Autodesk Inventor part; units mm, degrees
ref_plane "Flange Pattern Plane" through (19.05, 7.9375, -4.5466) normal (0, 1, 0) x (1, 0, 0)
ref_plane "YZ Plane" through (0, 0, 0) normal (1, 0, 0) x (0, 1, 0)
ref_plane "XZ Plane" through (0, 0, 0) normal (0, 1, 0) x (-1, 0, 0)
sketch "Sketch1" plane through (0, 0, 0) normal (0, 1, 0) x (-1, 0, 0)
  line L0 (-19.05, 0) -> (19.05, 0)
  line L1 (19.05, 0) -> (19.05, -12.7)
  line L2 (19.05, -12.7) -> (-19.05, -12.7)
  line L3 (-19.05, -12.7) -> (-19.05, 0)
  line L4 (19.05, 0) -> (-19.05, -12.7) construction
  point P0 (0, 0)
  point P1 (0, 0)
  dimension "d0" = 38.1
  dimension "d1" = 12.7
extrude "Plate1" add sketch "Sketch1" along normal blind 1.5875
sketch "Sketch2" plane through (17.4625, 0, -12.7) normal (1, 0, 0) x (0, 1, 0)
  line L0 (0, 12.7) -> (0, 0)
  line L1 (0, 0) -> (14.2875, 0)
  line L2 (14.2875, 0) -> (14.2875, 12.7)
  line L3 (14.2875, 12.7) -> (0, 12.7)
edge flange "Flanges" height 12.7 angle 90 thickness 1.5875 bend radius 0.7937 thickness toward (1, 0, 0) relief tear relief width 1.5875 relief depth 0.7937 corner gap 1.5875 corner form 0 edges at (19.05, 1.5875, -6.35) (-19.05, 1.5875, -6.35) wall of the first edge with corners at (17.4625, 0, 0) (17.4625, 0, -12.7) (17.4625, 14.2875, -12.7) (17.4625, 14.2875, 0)
bend "Bend1"
corner "Corner1"
sketch "Sketch3" plane through (19.05, 2.3813, -12.7) normal (1, 0, 0) x (0, 0, -1)
  line L0 (-8.1534, 7.8676) -> (-4.5466, 7.8676)
  line L1 (-4.0386, 7.3596) -> (-4.0386, 3.7529)
  line L2 (-4.5466, 3.2449) -> (-8.1534, 3.2449)
  line L3 (-8.6614, 3.7529) -> (-8.6614, 7.3596)
  arc A0 (-8.1534, 7.8676) -> (-8.6614, 7.3596) centre (-8.1534, 7.3596) ccw
  arc A1 (-4.0386, 7.3596) -> (-4.5466, 7.8676) centre (-4.5466, 7.3596) ccw
  arc A2 (-4.5466, 3.2449) -> (-4.0386, 3.7529) centre (-4.5466, 3.7529) ccw
  arc A3 (-8.6614, 3.7529) -> (-8.1534, 3.2449) centre (-8.1534, 3.7529) ccw
  line L4 (-12.7, 0) -> (-12.7, 11.9063) construction
  line L5 (-12.7, 11.9063) -> (0, 11.9063) construction
  line L6 (-8.1534, 7.3596) -> (-4.5466, 3.7529) construction
  point P0 (-12.7, -2.3812)
  point P1 (-4.0386, 3.2449)
  point P2 (-8.6614, 3.2449)
  point P3 (-6.35, 5.5563)
  dimension "d16" = 4.6228
  dimension "d17" = 0.508
  dimension "d20" = 6.35
  dimension "d21" = 6.35
extrude "Flange Stamp" cut sketch "Sketch3" against normal blind 1.5875
sketch "Sketch7" plane through (19.05, 2.3813, 0) normal (1, 0, 0) x (0, 0, -1)
  arc A0 (4.5466, 7.8676) -> (4.0386, 7.3596) centre (4.5466, 7.3596) ccw construction
  arc A1 (8.1534, 3.2449) -> (8.6614, 3.7529) centre (8.1534, 3.7529) ccw construction
  circle A2 centre (6.35, 5.5563) radius 2.1844
  line L0 (4.5466, 7.3596) -> (8.1534, 3.7529) construction
  point P0 (0, -2.3812)
  dimension "d46" = 4.3688
surface extrude "Flange Circle" sketch "Sketch7" against normal up to surface (1.5875 mm away) shown yes curves A2
ref_plane "Flange Pattern Plane" through (19.05, 7.9375, -4.5466) normal (0, 1, 0) x (1, 0, 0)
feature "Flange Pattern" [suppressed]
sketch "Sketch8" plane through (0, 0, 0) normal (0, -1, 0) x (1, 0, 0)
  line L0 (16.6687, 0) -> (-16.6687, 0) construction
  line L1 (14.5034, -4.0386) -> (10.8966, -4.0386)
  line L2 (10.3886, -4.5466) -> (10.3886, -8.1534)
  line L3 (10.8966, -8.6614) -> (14.5034, -8.6614)
  line L4 (15.0114, -8.1534) -> (15.0114, -4.5466)
  arc A0 (15.0114, -4.5466) -> (14.5034, -4.0386) centre (14.5034, -4.5466) ccw
  arc A1 (14.5034, -8.6614) -> (15.0114, -8.1534) centre (14.5034, -8.1534) ccw
  arc A2 (10.3886, -8.1534) -> (10.8966, -8.6614) centre (10.8966, -8.1534) ccw
  arc A3 (10.8966, -4.0386) -> (10.3886, -4.5466) centre (10.8966, -4.5466) ccw
  line L5 (14.5034, -4.5466) -> (10.8966, -8.1534) construction
  line L6 (19.05, 0) -> (19.05, -12.7) construction
  point P0 (0, 0)
  point P1 (10.3886, -8.6614)
  point P2 (15.0114, -8.6614)
  point P3 (12.7, -6.35)
  dimension "d49" = 4.6228
  dimension "d50" = 0.508
  dimension "d51" = 6.35
  dimension "d52" = 6.35
extrude "Body Stamp" cut sketch "Sketch8" against normal blind 1.5875
sketch "Sketch9" plane through (0, 0, 0) normal (0, -1, 0) x (1, 0, 0)
  arc A0 (15.0114, -4.5466) -> (14.5034, -4.0386) centre (14.5034, -4.5466) ccw construction
  arc A1 (10.3886, -8.1534) -> (10.8966, -8.6614) centre (10.8966, -8.1534) ccw construction
  line L0 (14.5034, -4.5466) -> (10.8966, -8.1534) construction
  circle A2 centre (12.7, -6.35) radius 2.1844
  point P0 (0, 0)
  dimension "d55" = 4.3688
surface extrude "Body Circle" sketch "Sketch9" against normal up to surface (1.5875 mm away) shown yes curves A2
feature "Body Pattern" [suppressed]
sketch "Arc Length" plane through (17.4625, 2.3813, 0) normal (0, 0, 1) x (1, 0, 0)
  line L0 (0, 0) -> (1.5875, 0) construction
  arc A0 (-0.7938, -0.7938) -> (0, 0) centre (-0.7937, 0) ccw construction
  line L1 (-0.7938, -2.3813) -> (-0.7938, -0.7938) construction
  arc A1 (-0.7938, -2.3813) -> (1.5875, 0) centre (-0.7937, 0) ccw construction
  point P0 (-17.4625, -2.3812)
  dimension "d85" = 3.7405
  dimension "d92" = 1.2468
sketch "Sketch13" plane through (19.05, 14.2875, 0) normal (1, 0, 0) x (0, 0, -1)
  line L0 (0, 0) -> (12.7, 0) construction
  line L1 (62.4078, 0) -> (63.4238, -1.016)
  line L2 (63.4238, -1.016) -> (64.4398, 0)
  line L3 (62.4078, 0) -> (64.4398, 0)
  line L4 (12.7, -11.9063) -> (0, -11.9062) construction
  line L5 (63.4238, -10.8903) -> (61.161, -13.1531)
  line L6 (61.161, -13.1531) -> (63.4238, -15.4159)
  line L7 (63.4238, -15.4159) -> (65.6866, -13.1531)
  line L8 (65.6866, -13.1531) -> (63.4238, -10.8903)
  line L9 (63.4238, -10.8903) -> (63.4238, -15.4159) construction
  line L10 (63.4238, -1.016) -> (63.4238, -10.8903) construction
  line L11 (0, -11.9062) -> (12.7, -11.9063) construction
  point P0 (0, -14.2875)
  dimension "d86" = 4.5256
  dimension "d88" = 1.016
  dimension "d91" = 1.016
  dimension "d102" = 63.4238
feature "Notch" [suppressed]
mirror "Notch Mirror" [suppressed]
pattern_linear "Notch Pattern" [suppressed]
chamfer "End Chamfer" distance 1.016 angle 45 4 edges at (-18.2563, 14.2875, -12.7) (18.2563, 14.2875, -12.7) (-18.2562, 14.2875, 0) (18.2562, 14.2875, 0)
sketch "Sketch14" plane through (-19.05, 2.3813, 431.8) normal (1, 0, 0) x (0, 0, -1)
  line L0 (431.8, 11.9063) -> (444.5, 11.9063) construction
  line L1 (431.8, 0) -> (431.8, 11.9063) construction
  line L2 (431.8, -2.3813) -> (444.5, -2.3813) construction
  line L3 (431.8, 11.9063) -> (444.5, 11.9063)
  line L4 (444.5, 11.9063) -> (444.5, -2.3813)
  line L5 (444.5, -2.3813) -> (431.8, -2.3813)
  line L6 (431.8, -2.3813) -> (431.8, 11.9063)
  point P0 (431.8, -2.3812)
  point P1 (382.0521, -1.9844)
extrude "Half Cut" cut sketch "Sketch14" along normal blind 25.4
sketch "Flange Pattern Sketch" plane through (19.05, 7.9375, -4.5466) normal (0, 1, 0) x (1, 0, 0)
  line L0 (0, 3.6068) -> (0, 0) construction
  line L1 (-45.8186, -4.5466) -> (8.2118, -4.5466) construction
  line L2 (0, 0) -> (-1.5875, 0) construction
  point P0 (-19.05, -4.5466)
  point P1 (0, 1.8034)
  point P2 (0, 14.5034)
  point P3 (0, 27.2034)
  point P4 (0, 39.9034)
  point P5 (0, 52.6034)
  point P6 (0, 65.3034)
  point P7 (0, 78.0034)
  point P8 (0, 90.7034)
  point P9 (0, 103.4034)
  point P10 (0, 116.1034)
  point P11 (0, 128.8034)
  point P12 (0, 141.5034)
  point P13 (0, 154.2034)
  point P14 (0, 166.9034)
  point P15 (0, 179.6034)
  point P16 (0, 192.3034)
  point P17 (0, 205.0034)
  point P18 (0, 217.7034)
  point P19 (0, 230.4034)
  point P20 (0, 243.1034)
  point P21 (0, 255.8034)
  point P22 (0, 268.5034)
  point P23 (0, 281.2034)
  point P24 (0, 293.9034)
  point P25 (0, 306.6034)
  point P26 (0, 319.3034)
  point P27 (0, 332.0034)
  point P28 (0, 344.7034)
  point P29 (0, 357.4034)
  point P30 (0, 370.1034)
  point P31 (0, 382.8034)
  point P32 (0, 395.5034)
  point P33 (0, 408.2034)
  point P34 (0, 420.9034)
  point P35 (0, 433.6034)
  dimension "d131" = 12.7
  dimension "d134" = 12.7
sketch "Body Pattern Sketch" plane through (0, 0, 0) normal (0, -1, 0) x (1, 0, 0)
  line L0 (16.6687, 0) -> (-16.6687, 0) construction
  line L1 (19.05, 0) -> (19.05, -12.7) construction
  circle A0 centre (12.7, -6.35) radius 2.1844 construction
  point P0 (0, 0)
  point P1 (12.7, -19.05)
  point P2 (12.7, -31.75)
  point P3 (12.7, -44.45)
  point P4 (12.7, -57.15)
  point P5 (12.7, -69.85)
  point P6 (12.7, -82.55)
  point P7 (12.7, -95.25)
  point P8 (12.7, -107.95)
  point P9 (12.7, -120.65)
  point P10 (12.7, -133.35)
  point P11 (12.7, -146.05)
  point P12 (12.7, -158.75)
  point P13 (12.7, -171.45)
  point P14 (12.7, -184.15)
  point P15 (12.7, -196.85)
  point P16 (12.7, -209.55)
  point P17 (12.7, -222.25)
  point P18 (12.7, -234.95)
  point P19 (12.7, -247.65)
  point P20 (12.7, -260.35)
  point P21 (12.7, -273.05)
  point P22 (12.7, -285.75)
  point P23 (12.7, -298.45)
  point P24 (12.7, -311.15)
  point P25 (12.7, -323.85)
  point P26 (12.7, -336.55)
  point P27 (12.7, -349.25)
  point P28 (12.7, -361.95)
  point P29 (12.7, -374.65)
  point P30 (12.7, -387.35)
  point P31 (12.7, -400.05)
  point P32 (12.7, -412.75)
  point P33 (12.7, -425.45)
  point P34 (12.7, -438.15)
  dimension "d62" = 12.7
  dimension "d65" = 12.7
  dimension "d139" = 12.7
equation "\"d1\" = 1.27 * Length"
equation "\"d18\" = Thickness"
equation "\"d53\" = Thickness"
equation "\"d89\" = Thickness"
equation "\"d2\" = Thickness"
equation "\"d3\" = BendReliefWidth"
equation "\"d4\" = BendReliefDepth"
equation "\"d5\" = MinimumRemnant"
equation "\"d6\" = TransitionRadius"
equation "\"d10\" = CornerReliefSize"
equation "\"d11\" = GapSize"
equation "\"d12\" = JacobiRadiusSize"
equation "\"BendRadius\" = Thickness"
equation "\"BendReliefWidth\" = Thickness"
equation "\"BendReliefDepth\" = 0.5 * Thickness"
equation "\"CornerReliefSize\" = 4 * Thickness"
equation "\"MinimumRemnant\" = 2 * Thickness"
equation "\"TransitionRadius\" = BendRadius"
equation "\"JacobiRadiusSize\" = BendRadius"
equation "\"GapSize\" = Thickness"
properties part number "Alu C 1x3x1x35"
The listing builds one solid part. Answer for the finished solid, in the listing's coordinates (mm). A direction names the side the tool comes from. Round coordinates to 2 decimals unless told otherwise and drop trailing zeros. Order: outer loops, then holes, each group sorted by start corner. A loop starts at its lowest first (then second) coordinate and runs counter-clockwise, first axis right, second up. Notation, with made-up numbers: (89, -12.5) -> (119, -12.5) arc R36 cw to (119, 22.5) -> close; hole circle Ø4 at (44, 8). An arc over 180 degrees is marked (long way). Answer as CSV lines item,"result". Start each with the question number.
(1) The part is cut by section B-B (z = -6). Determine the outline of the cut face in (x, y).
(2) The part is cut by section D-D (z = -9). Determine the outline of the cut face in (x, y).
(3) A tool of negligible diameter and unlimited length cuts with its end or side. For faces 5 (the face through (17.462, 11, -6)), 6 (the face through (10.389, 1, -6)), 7 (the face through (18, 8, -8.661)), 8 (the face through (18.27, 13.79, -0.52)), 9 (the face through (18.371, 0.716, -6.439)), from which of +Z, -Z, +X, -X, +Y, -Y can it reach the whole face along a straight path? Write none if from no direction.
(4) For a pull along Y with two mould halves and no side action, classify faces 1 (the face through (9, 0, -6)), 2 (the face through (18, 5.626, -6)), 3 (the face through (18, 8, -4.039)), 4 (the face through (9, 1.588, -6)) as +Y half, -Y half, draft (parallel to the pull), parting line (faces both ways), or undercut.
(5) The part is cut by section A-A (y = 7.25). Determine the outline of the cut face in (x, z), then the cut area to 3 significant figures.
(6) Find the intervals of material crossed by probe 1 along Z at (x, y) = (14, 0.5); probe 2 along X at (y, z) = (7, -4); probe 3 along Y at (x, z) = (13, -3.5), in increasing order. Write a range as from..to.
(7) Flat-ended cylindrical pins translate along their axes: pin 1 Ø6 at (y, z) = (8, -7) entering from -X; pin 2 Ø1 at (x, z) = (9, -10) entering from +Y; pin 3 Ø1.3 at (y, z) = (0.5, -7) entering from +X. Find the tip coordinate at first contact, or state that the pin passes through.
(8) The part is cut by section C-C (x = 11.25). Determine the outline of the cut face in (y, z), then the cut area to 3 significant figures.
Evaluation:
1,outline,"(6.35, 0) -> (10.39, 0) -> (10.39, 1.59) -> (6.35, 1.59) -> close; (15.01, 0) -> (16.67, 0) arc R2.38 ccw to (19.05, 2.38) -> (19.05, 5.63) -> (17.46, 5.63) -> (17.46, 2.38) arc R0.79 cw to (16.67, 1.59) -> (15.01, 1.59) -> close; (17.46, 10.25) -> (19.05, 10.25) -> (19.05, 14.29) -> (17.46, 14.29) -> close"
2,outline,"(6.35, 0) -> (16.67, 0) arc R2.38 ccw to (19.05, 2.38) -> (19.05, 14.29) -> (17.46, 14.29) -> (17.46, 2.38) arc R0.79 cw to (16.67, 1.59) -> (6.35, 1.59) -> close"
3,face 5,"+Z, -Z, -X, +Y"
3,face 6,"+Y, -Y"
3,face 7,"+X, -X"
3,face 8,"+Z, +X, -X, +Y"
3,face 9,"+Z, -Z, +X, -Y"
4,face 1,"-Y half"
4,face 2,"undercut"
4,face 3,"undercut"
4,face 4,"+Y half"
5,outline,"(17.46, -12.7) -> (19.05, -12.7) -> (19.05, -8.66) -> (17.46, -8.66) -> close; (17.46, -4.04) -> (19.05, -4.04) -> (19.05, 0) -> (17.46, 0) -> close"
5,area,"12.8 mm²"
6,probe 1,"-12.7..-8.66, -4.04..0"
6,probe 2,"17.46..19.05"
6,probe 3,"0..1.59"
7,pin 1,"x = 17.46"
7,pin 2,"y = 1.59"
7,pin 3,"x = 18.71"
8,outline,"(0, -12.7) -> (1.59, -12.7) -> (1.59, -8.66) -> (0, -8.66) -> close; (0, -4.04) -> (1.59, -4.04) -> (1.59, 0) -> (0, 0) -> close"
8,area,"12.8 mm²"
